For this review, take the finished solid that the model builds, in its own axes (mm). Give positions to 0.01 mm unless a question says otherwise; leave off trailing zeros. Loops run counter-clockwise (first coordinate to the right, second up) from the corner with the lowest first, then second, coordinate; pieces in that order, holes last.
```python
from build123d import *

# Parameters (mm, degrees)
SKETCH1_R               = 4.7625
SKETCH1_R_2             = 3.018976491
BOSS_EXTRUDE1_DEPTH     = 65
SKETCH5_W               = 36.473052953
SKETCH5_H               = 81.397778837
CUT_EXTRUDE2_DEPTH      = 5.7625
CUT_EXTRUDE2_DEPTH_BACK = 5.7625
SKETCH6_W               = 37.230077322
SKETCH6_H               = 44.032609969
CUT_EXTRUDE3_DEPTH      = 5.7625
CUT_EXTRUDE3_DEPTH_BACK = 5.7625


with BuildPart() as part:
    # Sketch1 → Boss-Extrude1 (new body, symmetric)
    with BuildSketch(Plane(origin=(0, 0, 0), x_dir=(1, 0, 0), z_dir=(0, 1, 0))):
        Circle(SKETCH1_R)
        Circle(SKETCH1_R_2, mode=Mode.SUBTRACT)
    extrude(amount=BOSS_EXTRUDE1_DEPTH, both=True)

    # Sketch5 → Cut-Extrude2 (cut, two sides)
    with BuildSketch(Plane(origin=(0, 0, 0), x_dir=(0, 0, -1), z_dir=(1, 0, 0))) as cut_extrude2_sk:
        with Locations((-2.67750977, 45.698889419)):
            Rectangle(SKETCH5_W, SKETCH5_H)
    extrude(amount=CUT_EXTRUDE2_DEPTH, mode=Mode.SUBTRACT)
    extrude(cut_extrude2_sk.sketch, amount=-CUT_EXTRUDE2_DEPTH_BACK, mode=Mode.SUBTRACT)

    # Sketch6 → Cut-Extrude3 (cut, two sides)
    with BuildSketch(Plane(origin=(0, 0, 0), x_dir=(0, 0, -1), z_dir=(1, 0, 0))) as cut_extrude3_sk:
        with Locations((-3.171451031, -53.016304985)):
            Rectangle(SKETCH6_W, SKETCH6_H)
    extrude(amount=CUT_EXTRUDE3_DEPTH, mode=Mode.SUBTRACT)
    extrude(cut_extrude3_sk.sketch, amount=-CUT_EXTRUDE3_DEPTH_BACK, mode=Mode.SUBTRACT)


solid = part.part
```
Item 1: Take a section at A-A on z = 0. Give the boundary of the cut face in (x, y).
Answer:
outline: (-4.76, -31) - (-3.02, -31) - (-3.02, 5) - (-4.76, 5) - close; (3.02, -31) - (4.76, -31) - (4.76, 5) - (3.02, 5) - close
Item 2: Take a section at B-B on x = 0. Give the boundary of the cut face in (y, z).
Answer:
outline: (-31, -4.76) - (5, -4.76) - (5, -3.02) - (-31, -3.02) - close; (-31, 3.02) - (5, 3.02) - (5, 4.76) - (-31, 4.76) - close
Item 3: The part is to be moulded in two halves that separate along X. For faces 1 (the cylindrical face through (2.88, -13.25, -0.91)), 2 (the cylindrical face through (-3.78, -12.75, 2.9)), 3 (the flat face through (3.1, -31, -1)), say which applies: released by +X, released by -X, zero draft, split by the parting line, or undercut.
Answer:
face 1: undercut
face 2: split by the parting line
face 3: zero draft
Item 4: Take a section at C-C on y = -27. Give the boundary of the cut face in (x, z) (1 decimal), and give its area (3 significant figures).
Answer:
outline: circle Ø9.5 at (0, 0); hole circle Ø6 at (0, 0)
area: 42.6 mm2
Item 5: For L1, parallel to X at y = -9, z = 0; L2, parallel to Z at x = -1.5, y = -8.5, list the stretches that pass through material, from the lowest coordinate up.
Answer:
L1: x = -4.76 to -3.02, 3.02 to 4.76
L2: z = -4.52 to -2.62, 2.62 to 4.52
Item 6: Clearance check with flat-ended pins moving along their axes: pin 1 Ø5 at (x, y) = (-3.5, -10.5) entering from +Z; pin 2 Ø2 at (y, z) = (-22.5, -1.5) entering from -X. State where each tip first meets the part, or that it passes through.
Answer:
pin 1: stops at z = 4.66
pin 2: stops at x = -4.74
Item 7: Take a section at D-D on z = 4.25. Give the boundary of the cut face in (x, y).
Answer:
outline: (-2.15, -31) - (2.15, -31) - (2.15, 5) - (-2.15, 5) - close
